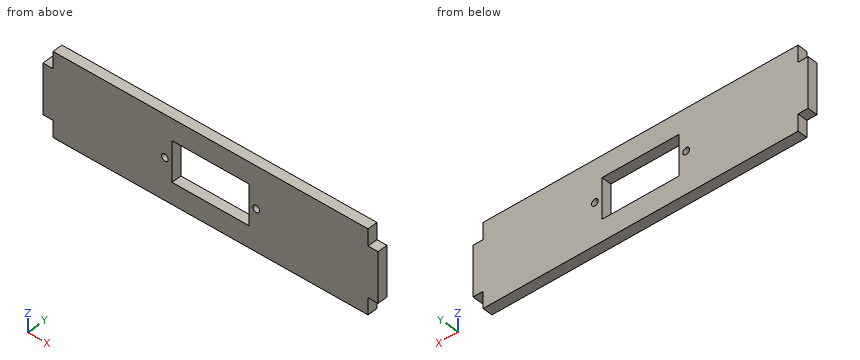
from build123d import *

# Parameters (mm, degrees)
BOSS_EXTRUDE1_DEPTH = 3
SKETCH2_R           = 1
SKETCH2_W           = 23
SKETCH2_H           = 12.1
CUT_EXTRUDE1_DEPTH  = 23.3


with BuildPart() as part:
    # Sketch1 → Boss-Extrude1 (new body)
    with BuildSketch(Plane(origin=(0, 0, 0), x_dir=(1, 0, 0), z_dir=(0, 1, 0))):
        Polygon((47, -7.5), (50, -7.5), (50, 7.5), (47, 7.5), (47, 12.5), (-47, 12.5), (-47, 7.5), (-50, 7.5), (-50, -7.5), (-47, -7.5), (-47, -12.5), (47, -12.5), align=None)
    extrude(amount=BOSS_EXTRUDE1_DEPTH)

    # Sketch2 → Cut-Extrude1 (cut)
    with BuildSketch(Plane(origin=(0, 3, 0), x_dir=(1, 0, 0), z_dir=(0, 1, 0))):
        with Locations(Location((-13.625, 0, 0), (0, 0, 270))):
            Circle(SKETCH2_R)
        with Locations(Location((13.625, 0, 0), (0, 0, 270))):
            Circle(SKETCH2_R)
        Rectangle(SKETCH2_W, SKETCH2_H)
    extrude(amount=-CUT_EXTRUDE1_DEPTH, mode=Mode.SUBTRACT)


solid = part.part
Work out the finished part from the listing and answer in its coordinate system (mm). Coordinates: 2 decimals unless noted, no trailing zeros. Write each loop counter-clockwise with the first axis right and the second up, starting at its lowest first coordinate (ties: lowest second). Pieces come first, ordered by that corner, then holes. Notation, with made-up numbers: M -37.5,82.25 L -25.5,82.25 A17 cw -25.5,109.25 Z; hole C -8.75,5 d2. An arc over 180 degrees is marked long. Write item = value, one per line.
1. The part is cut by section B-B (z = 0). Determine the outline of the cut face in (x, y) (3 decimals).
Solution:
outline = M -50,0 L -14.625,0 L -14.625,3 L -50,3 Z; M -12.625,0 L -11.5,0 L -11.5,3 L -12.625,3 Z; M 11.5,0 L 12.625,0 L 12.625,3 L 11.5,3 Z; M 14.625,0 L 50,0 L 50,3 L 14.625,3 Z
2. The part is cut by section A-A (z = 4). Determine the outline of the cut face in (x, y), then the cut area to 3 significant figures.
Solution:
outline = M -50,0 L -11.5,0 L -11.5,3 L -50,3 Z; M 11.5,0 L 50,0 L 50,3 L 11.5,3 Z
area = 231 mm2
3. Flat-ended cylindrical pins translate along their axes: pin 1 (2.5 mm diameter, centred on x = -13.625, z = 0, fed in from -Y); pin 2 (1.5 mm diameter, centred on y = 1, z = 11, fed in from -X); pin 3 (1 mm diameter, centred on y = 2, z = 8.5, fed in from +X); pin 4 (0.9 mm diameter, centred on x = -48, y = 1.5, fed in from +Z). Find the tip coordinate at first contact, or state that the pin passes through.
Solution:
pin_1 = 0
pin_2 = -47
pin_3 = 47
pin_4 = 7.5
4. Straight lines are drawn through the part: line 1 (X direction, y = 2.45, z = 0) (3 decimals); line 2 (Z direction, x = 6, y = 0.8); line 3 (X direction, y = 1.05, z = -0.25). For each, find the intervals that lie inside material, in ascending order. Write a range as from..to.
Solution:
line_1 = -50..-14.625, -12.625..-11.5, 11.5..12.625, 14.625..50
line_2 = -12.5..-6.05, 6.05..12.5
line_3 = -50..-14.59, -12.66..-11.5, 11.5..12.66, 14.59..50
5. The part is cut by section D-D (z = 9.5). Determine the outline of the cut face in (x, y), then the cut area to 3 significant figures.
Solution:
outline = M -47,0 L 47,0 L 47,3 L -47,3 Z
area = 282 mm2
6. The part is cut by section C-C (y = 1.6). Determine the outline of the cut face in (x, z) (3 decimals), then the cut area to 3 significant figures.
Solution:
outline = M -50,-7.5 L -47,-7.5 L -47,-12.5 L 47,-12.5 L 47,-7.5 L 50,-7.5 L 50,7.5 L 47,7.5 L 47,12.5 L -47,12.5 L -47,7.5 L -50,7.5 Z; hole C -13.625,0 d2; hole M -11.5,-6.05 L 11.5,-6.05 L 11.5,6.05 L -11.5,6.05 Z; hole C 13.625,0 d2
area = 2,160 mm2
